Part print with two shaded views. Sizes in mm from the minimum x, y, z corner. A direction names the side the tool comes from. Round coordinates to 2 decimals unless told otherwise and drop trailing zeros. Order: outer loops, then holes, each group sorted by start corner. A loop starts at its lowest first (then second) coordinate and runs counter-clockwise, first axis right, second up. Notation, with made-up numbers: (10, 13) - (48, 13) arc R8 cw to (48, 27) - close; hole circle Ø2 at (-23.5, 71). An arc over 180 degrees is marked (long way). Write item = value, one per line.
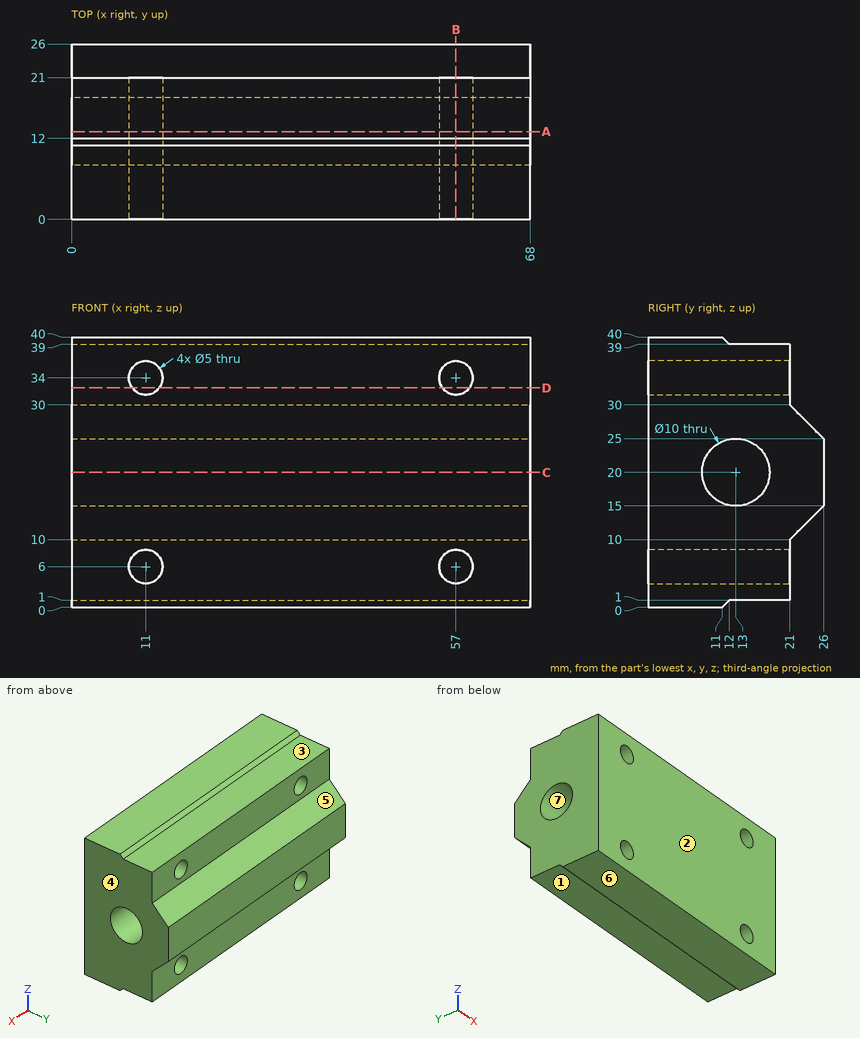
1) Cut at B-B (x = 57). Give the number of separate pieces and of enclosed holes in the cut face.
Conclusion:
separate_pieces = 3
enclosed_holes = 1
2) Mould opens along Z. For the marked faces 4, 5, 6 and 7 say: +Z half, -Z half, draft (parallel to the pull), parting line (faces both ways), or undercut.
Conclusion:
face_4 = draft
face_5 = +Z half
face_6 = -Z half
face_7 = undercut
3) Cut at A-A (y = 13). Write the cut outline in (x, z), and give its area (3 significant figures).
Conclusion:
outline = (0, 1) - (68, 1) - (68, 15) - (0, 15) - close; (0, 25) - (68, 25) - (68, 39) - (0, 39) - close; hole circle Ø5 at (11, 6); hole circle Ø5 at (11, 34); hole circle Ø5 at (57, 6); hole circle Ø5 at (57, 34)
area = 1,830 mm^2
4) Cut at D-D (z = 32.5). Write the cut outline in (x, y), and give its area (3 significant figures).
Conclusion:
outline = (0, 0) - (9, 0) - (9, 21) - (0, 21) - close; (13, 0) - (55, 0) - (55, 21) - (13, 21) - close; (59, 0) - (68, 0) - (68, 21) - (59, 21) - close
area = 1,260 mm^2
5) Wall check: line 1 along Z through (x, y) = (11, 7.25); line 2 along X through (y, z) = (16, 6); line 3 along Z through (x, y) = (57, 10.75) (1 decimal). Give the ranges that are in metal, low to high.
Conclusion:
line_1 = 0 to 3.5, 8.5 to 31.5, 36.5 to 40
line_2 = 0 to 8.5, 13.5 to 54.5, 59.5 to 68
line_3 = 0 to 3.5, 8.5 to 15.5, 24.5 to 31.5, 36.5 to 40
6) 3-axis set-ups, long thin cutter, end or side, ignore diameter. For the marked faces 1, 2 and 3: which of +Z, -Z, +X, -X, +Y, -Y reach the whole face in a straight line?
Conclusion:
face_1 = -Z, +X, -X, +Y
face_2 = +Z, -Z, +X, -X, -Y
face_3 = +Z, +X, -X, +Y
7) Cut at C-C (z = 20). Write the cut outline in (x, y), and give its area (3 significant figures).
Conclusion:
outline = (0, 0) - (68, 0) - (68, 8) - (0, 8) - close; (0, 18) - (68, 18) - (68, 26) - (0, 26) - close
area = 1,090 mm^2
8) Flat gauge pins, fed straight in: pin 1 Ø4.5 at (x, y) = (30.5, 18) entering from +Z; pin 2 Ø7 at (x, y) = (25.5, 17) entering from -Z; pin 3 Ø7 at (x, z) = (23.5, 7.5) entering from +Y; pin 4 Ø4 at (x, z) = (57, 34) entering from -Y. Where does each tip first touch, or does it go through?
Conclusion:
pin_1 = 39
pin_2 = 1
pin_3 = 22
pin_4 = through
